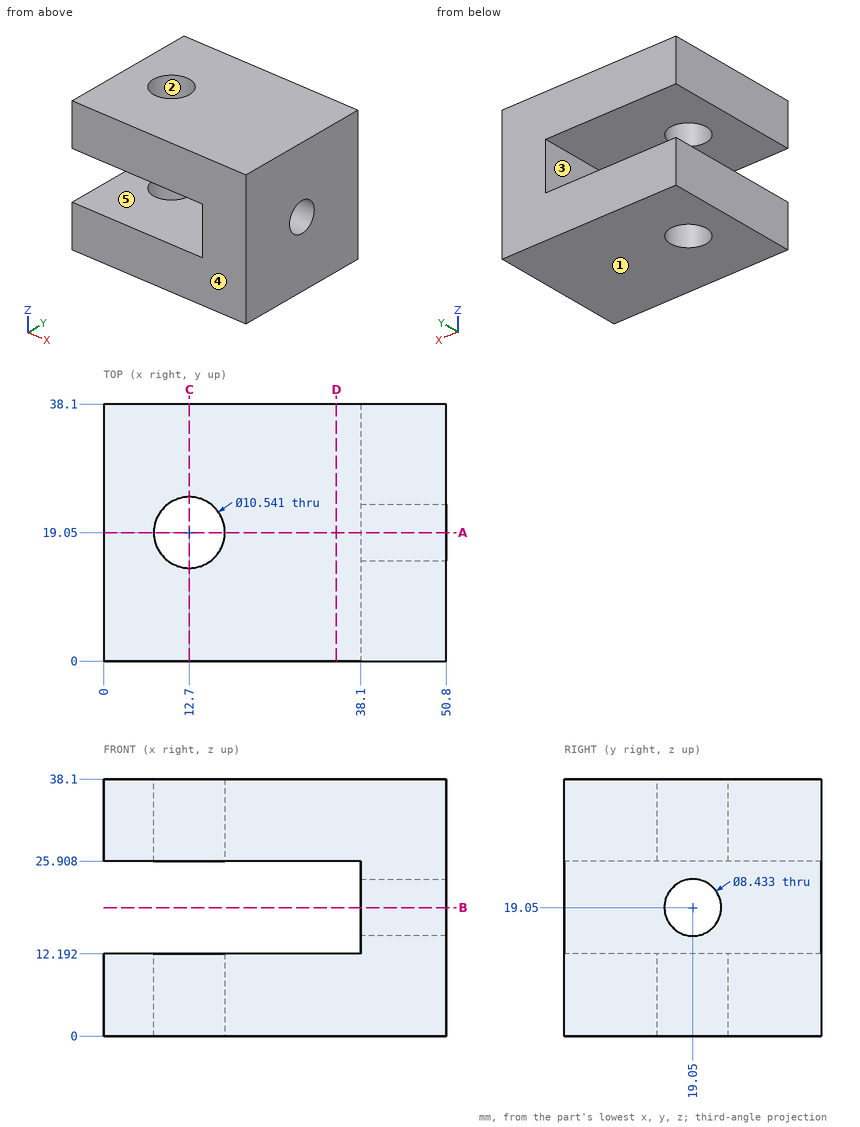
Here's the drawing with two shaded views (mm, measured from the low corner). I have some questions. A direction names the side the tool comes from. Round coordinates to 2 decimals unless told otherwise and drop trailing zeros. Write each loop counter-clockwise with the first axis right and the second up, starting at its lowest first coordinate (ties: lowest second). Pieces come first, ordered by that corner, then holes. Notation, with made-up numbers: M 52.5,-20.5 L 111.5,-20.5 A5 ccw 111.5,-12.5 Z; hole C 67,27 d5. An arc over 180 degrees is marked long. Write each question's results on one line, items separated by ' | '. Start each with the question number.
1. Imagine slicing it at C-C on x = 12.7. List the corners of the cut face in (y, z) for me, and give its area (3 significant figures).
2. Thinking about a two-plate mould opening in Z: for the marked faces 1, 2 and 3, which applies, +Z half, -Z half, draft (parallel to the pull), parting line (faces both ways), or undercut?
3. I need wall thicknesses on L1, parallel to Z at x = 44, y = 19; L2, parallel to Y at x = 12.7, z = 34.25. Which ranges of each line are inside material? Lowest first, please. Write a range as from..to.
4. I'm going to push flat-ended pins straight in: pin 1 Ø3 at (x, z) = (21, 7.5) entering from -Y; pin 2 Ø7 at (y, z) = (18, 22) entering from -X; pin 3 Ø8.5 at (x, y) = (12.7, 19.05) entering from -Z. Where does each tip first touch, or does it pass through?
5. On a 3-axis mill with a long thin cutter (end or side, diameter ignored), from which of +Z, -Z, +X, -X, +Y, -Y can I reach the whole of each face in a straight line? I mean the marked faces 4 and 5. Say none if no direction works.
6. Imagine slicing it at D-D on x = 34.5. List the corners of the cut face in (y, z) for me, and give its area (3 significant figures).
7. Imagine slicing it at B-B on z = 19.05. List the corners of the cut face in (x, y) for me.
8. Imagine slicing it at A-A on y = 19.05. List the corners of the cut face in (x, z) for me, and give its area (3 significant figures).
Result sheet:
1) outline: M 0,0 L 13.78,0 L 13.78,12.19 L 0,12.19 Z; M 0,25.91 L 13.78,25.91 L 13.78,38.1 L 0,38.1 Z; M 24.32,0 L 38.1,0 L 38.1,12.19 L 24.32,12.19 Z; M 24.32,25.91 L 38.1,25.91 L 38.1,38.1 L 24.32,38.1 Z | area: 672 mm^2
2) face 1: -Z half | face 2: draft | face 3: undercut
3) L1: z = 0..14.83, 23.27..38.1 | L2: y = 0..13.78, 24.32..38.1
4) pin 1: stops at y = 0 | pin 2: stops at x = 38.1 | pin 3: passes through
5) face 4: +Z, -Z, +X, -X, -Y | face 5: -X, +Y, -Y
6) outline: M 0,0 L 38.1,0 L 38.1,12.19 L 0,12.19 Z; M 0,25.91 L 38.1,25.91 L 38.1,38.1 L 0,38.1 Z | area: 929 mm^2
7) outline: M 38.1,0 L 50.8,0 L 50.8,14.83 L 38.1,14.83 Z; M 38.1,23.27 L 50.8,23.27 L 50.8,38.1 L 38.1,38.1 Z
8) outline: M 0,0 L 7.43,0 L 7.43,12.19 L 0,12.19 Z; M 0,25.91 L 7.43,25.91 L 7.43,38.1 L 0,38.1 Z; M 17.97,0 L 50.8,0 L 50.8,14.83 L 38.1,14.83 L 38.1,12.19 L 17.97,12.19 Z; M 17.97,25.91 L 38.1,25.91 L 38.1,23.27 L 50.8,23.27 L 50.8,38.1 L 17.97,38.1 Z | area: 1,050 mm^2
